```python
from build123d import *

# Parameters (mm, degrees)
BOSS_EXTRUDE1_DEPTH = 4.12
SKETCH2_R           = 2.55
CUT_EXTRUDE1_DEPTH  = 5.12


with BuildPart() as part:
    # Sketch1 → Boss-Extrude1 (new body)
    with BuildSketch(Plane.XY):
        Polygon((0, 0), (0, 60), (20, 60), (60, 20), (60, 0), align=None)
    extrude(amount=BOSS_EXTRUDE1_DEPTH)

    # Sketch2 → Cut-Extrude1 (cut, through all)
    with BuildSketch(Plane.XY.offset(4.12)):
        with Locations((10, 10)):
            Circle(SKETCH2_R)
        with Locations((30, 10)):
            Circle(SKETCH2_R)
        with Locations((50, 10)):
            Circle(SKETCH2_R)
        with Locations((10, 30)):
            Circle(SKETCH2_R)
        with Locations((10, 50)):
            Circle(SKETCH2_R)
    extrude(amount=-CUT_EXTRUDE1_DEPTH, mode=Mode.SUBTRACT)


solid = part.part
```
Read the model definition and answer for the solid it produces. Units are mm, in the model's axes. Coordinates: 2 decimals unless noted, no trailing zeros. Loops run counter-clockwise (first coordinate to the right, second up) from the corner with the lowest first, then second, coordinate; pieces in that order, holes last. Notation, with made-up numbers: (27, 11.25) - (60, 11.25) arc R14 cw to (60, 25.25) - close; hole circle Ø5 at (-2, -32). An arc over 180 degrees is marked (long way). Answer in a Markdown table with one row per item.
1. Find section C-C, the plane z = 2.2. Write down the section's boundary in (x, y), then the cut area to 3 significant figures.
Conclusion:
| item | result |
|---|---|
| outline | (0, 0) - (60, 0) - (60, 20) - (20, 60) - (0, 60) - close; hole circle Ø5.1 at (10, 10); hole circle Ø5.1 at (10, 30); hole circle Ø5.1 at (10, 50); hole circle Ø5.1 at (30, 10); hole circle Ø5.1 at (50, 10) |
| area | 2,700 mm² |
2. Determine the mould class of faces 1 (the face through (40, 40, 2)), 2 (the face through (10, 60, 2)), 3 (the face through (9.67, 52.53, 2.09)), 4 (the face through (0, 30, 2)) for opening direction X: +X half, -X half, draft (parallel to the pull), parting line (faces both ways), or undercut.
Conclusion:
| item | result |
|---|---|
| face 1 | +X half |
| face 2 | draft |
| face 3 | undercut |
| face 4 | -X half |
3. Find section D-D, the plane x = 50. Write down the section's boundary in (y, z), then the cut area to 3 significant figures.
Conclusion:
| item | result |
|---|---|
| outline | (0, 0) - (7.45, 0) - (7.45, 4.12) - (0, 4.12) - close; (12.55, 0) - (30, 0) - (30, 4.12) - (12.55, 4.12) - close |
| area | 103 mm² |
4. Find section A-A, the plane x = 10. Write down the section's boundary in (y, z), then the cut area to 3 significant figures.
Conclusion:
| item | result |
|---|---|
| outline | (0, 0) - (7.45, 0) - (7.45, 4.12) - (0, 4.12) - close; (12.55, 0) - (27.45, 0) - (27.45, 4.12) - (12.55, 4.12) - close; (32.55, 0) - (47.45, 0) - (47.45, 4.12) - (32.55, 4.12) - close; (52.55, 0) - (60, 0) - (60, 4.12) - (52.55, 4.12) - close |
| area | 184 mm² |
5. Straight lines are drawn through the part: line 1 (Y direction, x = 10, z = 1.5); line 2 (X direction, y = 50.5, z = 0.2); line 3 (Y direction, x = 29, z = 1.2). For each, find the intervals that lie inside material, in ascending order.
Conclusion:
| item | result |
|---|---|
| line 1 | y = 0 to 7.45, 12.55 to 27.45, 32.55 to 47.45, 52.55 to 60 |
| line 2 | x = 0 to 7.5, 12.5 to 29.5 |
| line 3 | y = 0 to 7.65, 12.35 to 51 |
